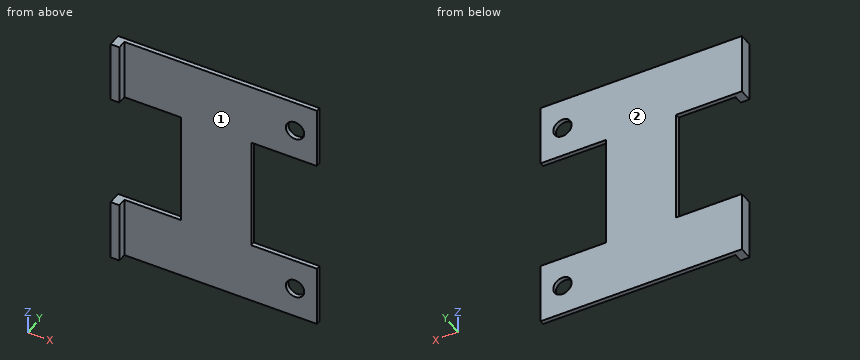
from build123d import *

# Parameters (mm, degrees)
SKETCH1_R           = 2.1
BOSS_EXTRUDE1_DEPTH = 1
SKETCH2_W           = 2
SKETCH2_H           = 14
BOSS_EXTRUDE2_DEPTH = 2


with BuildPart() as part:
    # Sketch1 → Boss-Extrude1 (new body)
    with BuildSketch(Plane(origin=(0, 0, 0), x_dir=(1, 0, 0), z_dir=(0, 1, 0))):
        Polygon((-30.551614771, -125.360414745), (-76.551614771, -125.360414745), (-76.551614771, -139.360414745), (-61.551614771, -139.360414745), (-61.551614771, -165.360414745), (-76.551614771, -165.360414745), (-76.551614771, -179.360414745), (-30.551614771, -179.360414745), (-30.551614771, -165.360414745), (-45.551614771, -165.360414745), (-45.551614771, -139.360414745), (-30.551614771, -139.360414745), align=None)
        with Locations((-35.551614771, -132.360414745)):
            Circle(SKETCH1_R, mode=Mode.SUBTRACT)
        with Locations((-35.551614771, -172.360414745)):
            Circle(SKETCH1_R, mode=Mode.SUBTRACT)
    extrude(amount=BOSS_EXTRUDE1_DEPTH)

    # Sketch2 → Boss-Extrude2 (add)
    with BuildSketch(Plane(origin=(0, 0, 0), x_dir=(-1, 0, 0), z_dir=(0, -1, 0))):
        with Locations((75.551614771, -172.360414745)):
            Rectangle(SKETCH2_W, SKETCH2_H)
        with Locations((75.551614771, -132.360414745)):
            Rectangle(SKETCH2_W, SKETCH2_H)
    extrude(amount=BOSS_EXTRUDE2_DEPTH)


solid = part.part
The listing builds one solid part. Answer for the finished solid, in the listing's coordinates (mm). Face numbers are marked on the shaded views. A direction names the side the tool comes from. Give positions to 0.01 mm unless a question says otherwise; leave off trailing zeros. Write each loop counter-clockwise with the first axis right and the second up, starting at its lowest first coordinate (ties: lowest second). Pieces come first, ordered by that corner, then holes.
1) Section B-B (y = -0.5) is taken. Write down the section's boundary in (x, z), and give its area (3 significant figures).
2) Section A-A (x = -73) is taken. Write down the section's boundary in (y, z).
3) A tool of negligible diameter and unlimited length cuts with its end or side. For the marked faces 1 and 2, from which of +Z, -Z, +X, -X, +Y, -Y can it reach the whole face along a straight path? Write none if from no direction.
4) Find the intervals of material crossed by L1, parallel to Y at x = -44.5, z = 168; L2, parallel to X at y = -0.9, z = 177; L3, parallel to X at y = 0.5, z = 156, in increasing order.
5) Section C-C (z = 147.5) is taken. Write down the section's boundary in (x, y).
6) Given P1, Ø13, axis at x = -60, z = 147, coming from the -Y side; P2, Ø0.6, axis at y = -0.5, z = 129, coming from the +X side; P3, Ø0.8, axis at y = 0.5, z = 156.5, coming from the -X side; P4, Ø2.5, axis at x = -35.55, z = 172.36, coming from the -Y side, each flat-ended and moving along its own axis, determine where each tip first touches the part or whether it passes through.
7) Section D-D (x = -58.5) is taken. Write down the section's boundary in (y, z).
Response:
1. outline: (-76.55, 125.36) - (-74.55, 125.36) - (-74.55, 139.36) - (-76.55, 139.36) - close; (-76.55, 165.36) - (-74.55, 165.36) - (-74.55, 179.36) - (-76.55, 179.36) - close
1. area: 56.0 mm2
2. outline: (0, 125.36) - (1, 125.36) - (1, 139.36) - (0, 139.36) - close; (0, 165.36) - (1, 165.36) - (1, 179.36) - (0, 179.36) - close
3. face 1: +Z, -Z, +X, -Y
3. face 2: +Z, -Z, +X, -X, +Y
4. L1: y = 0 to 1
4. L2: x = -76.55 to -74.55
4. L3: x = -61.55 to -45.55
5. outline: (-61.55, 0) - (-45.55, 0) - (-45.55, 1) - (-61.55, 1) - close
6. P1: stops at y = 0
6. P2: stops at x = -74.55
6. P3: stops at x = -61.55
6. P4: passes through
7. outline: (0, 125.36) - (1, 125.36) - (1, 179.36) - (0, 179.36) - close
